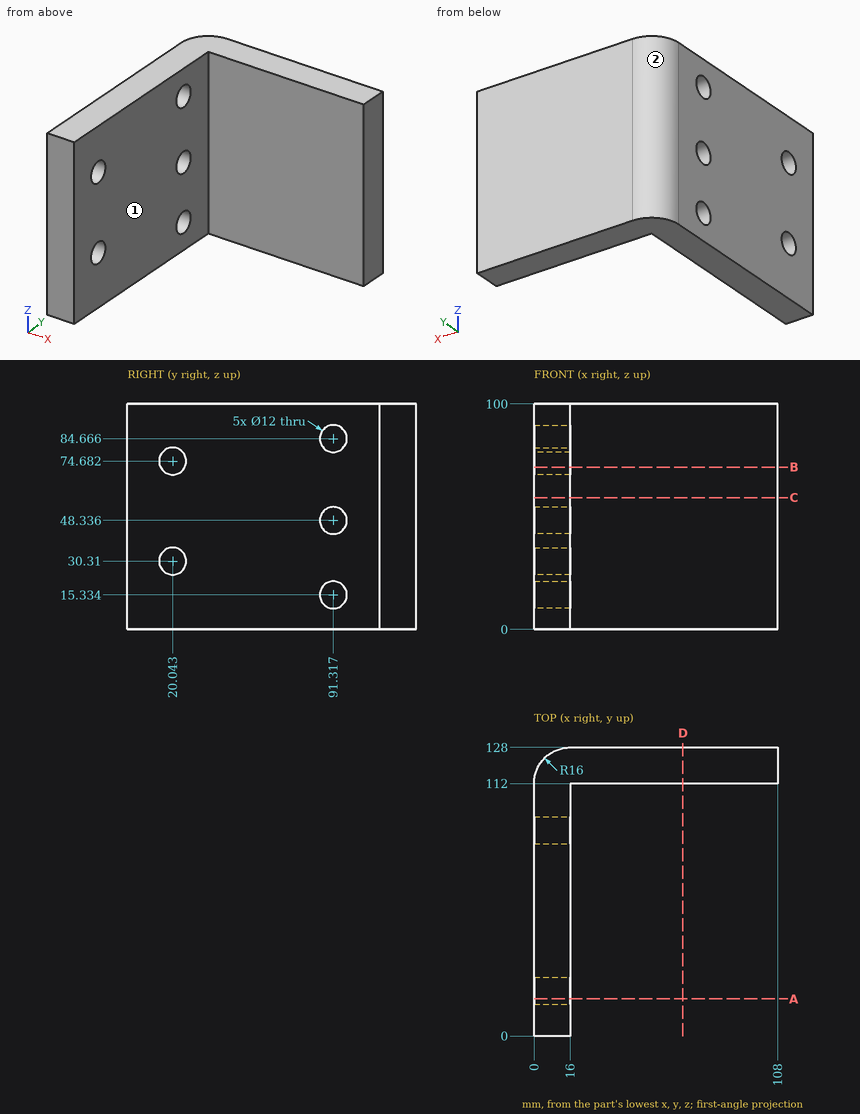
Geometry: see drawing. Coordinates: mm, zero at the bounding-box minimum. A direction names the side the tool comes from. Give positions to 0.01 mm unless a question says otherwise; leave off trailing zeros. Write each loop counter-clockwise with the first axis right and the second up, starting at its lowest first coordinate (ties: lowest second). Pieces come first, ordered by that corner, then holes. Notation, with made-up numbers: M 69.25,50 L 79.25,50 A26 cw 79.25,66 Z; hole C -36.75,82.5 d11. An arc over 180 degrees is marked long. Answer in a Markdown table with one row per item. Add a question column.
(1) Reachability of the marked faces 1 and 2 from +Z, -Z, +X, -X, +Y, -Y: full face, straight path, thin tool, end or side. Return the list, or none.
(2) Section D-D on x = 66. Return loops of the section in (y, z), and give its area (3 significant figures).
(3) Section B-B on z = 72. Return loops of the section in (x, y).
(4) Section C-C on z = 58.5. Return loops of the section in (x, y).
(5) Section A-A on y = 16.5. Return loops of the section in (x, z) (1 decimal).
(6) First-contact query: pin 1 (4 mm diameter, centred on y = 21.5, z = 34.5, fed in from +X). Flat tip, straight axial feed; report the tip coordinate or a pass-through.
(7) Ray query, line 1 (X direction, y = 100.5, z = 47.5); line 2 (Y direction, x = 48.5, z = 43); line 3 (Y direction, x = 5, z = 46) (1 decimal). Return the intervals inside material, ascending.
Result set:
| question | item | result |
|---|---|---|
| 1 | face 1 | +Z, -Z, +X, -Y |
| 1 | face 2 | +Z, -Z, -X, +Y |
| 2 | outline | M 112,0 L 128,0 L 128,100 L 112,100 Z |
| 2 | area | 1,600 mm^2 |
| 3 | outline | M 0,0 L 16,0 L 16,14.68 L 0,14.68 Z; M 0,25.41 L 16,25.41 L 16,112 L 108,112 L 108,128 L 16,128 A16 ccw 0,112 Z |
| 4 | outline | M 0,0 L 16,0 L 16,112 L 108,112 L 108,128 L 16,128 A16 ccw 0,112 Z |
| 5 | outline | M 0,0 L 16,0 L 16,25.5 L 0,25.5 Z; M 0,35.2 L 16,35.2 L 16,69.8 L 0,69.8 Z; M 0,79.5 L 16,79.5 L 16,100 L 0,100 Z |
| 6 | pin 1 | stops at x = 16 |
| 7 | line 1 | x = 0 to 16 |
| 7 | line 2 | y = 112 to 128 |
| 7 | line 3 | y = 0 to 85.8, 96.8 to 123.6 |
